Autodesk Inventor part; units mm, degrees
ref_plane "YZ Plane" through (0, 0, 0) normal (1, 0, 0) x (0, 1, 0)
ref_plane "XZ Plane" through (0, 0, 0) normal (0, 1, 0) x (-1, 0, 0)
ref_plane "XY Plane" through (0, 0, 0) normal (0, 0, 1) x (1, 0, 0)
sketch "Boceto1" plane through (0, 0, 0) normal (0, 0, 1) x (1, 0, 0)
  line L0 (220, 79) -> (220, 30)
  line L1 (229.5, 46) -> (229.5, 75)
  line L2 (235.5, 75) -> (235.5, 46)
  line L3 (229.5, -15) -> (229.5, 14)
  line L4 (235.5, 14) -> (235.5, -15)
  circle A0 centre (222.4918, -17.5) radius 1.6
  circle A1 centre (222.4918, 27.5) radius 1.6
  circle A2 centre (245.5, 27.5) radius 1.6
  circle A3 centre (245.5, -17.5) radius 1.6
  circle A4 centre (222.4918, 80) radius 1.6
  circle A5 centre (245.5, 75.9891) radius 1.6
  line L5 (220, 30) -> (220, -25)
  line L6 (229.5, 75) -> (230.4, 75)
  line L7 (231.4, 46) -> (229.5, 46)
  line L8 (220, -25) -> (227, -25)
  line L9 (238, -25) -> (240, -25)
  line L10 (231.4, -15) -> (229.5, -15)
  line L11 (229.5, 14) -> (231.4, 14)
  line L12 (230.4, 75) -> (235.5, 75)
  line L13 (231.4, 46) -> (235.5, 46)
  line L14 (231.4, 14) -> (235.5, 14)
  line L15 (231.4, -15) -> (235.5, -15)
  line L16 (227, -25) -> (238, -25)
  line L17 (245, 85) -> (220, 85)
  line L18 (220, 79) -> (220, 85)
  line L19 (251, 85) -> (251, -25)
  line L20 (240, -25) -> (251, -25)
  line L21 (245, 85) -> (251, 85)
  point P0 (0, 0)
  point P1 (245, -15)
  point P2 (245, 75)
  dimension "d2" = 6
  dimension "d3" = 9.5
  dimension "d4" = 6
  dimension "d5" = 9.5
  dimension "d6" = 29
  dimension "d9" = 9.0109
  dimension "d10" = 5
  dimension "d11" = 10
  dimension "d14" = 25.5
  dimension "d15" = 25.5
  dimension "d16" = 25.5
extrude "Extrusión1" add sketch "Boceto1" along normal blind 5
fillet "Empalme1" radius 1 2 edges at (251, 85, 2.5) (220, 85, 2.5)
fillet "Empalme2" radius 5 1 edges at (251, -25, 2.5)
properties part number "suplemento cojinete tapa"
Design review of the part built by this model. Coordinates are the model's own, in mm. A direction names the side the tool comes from. Give positions to 0.01 mm unless a question says otherwise; leave off trailing zeros. Write each loop counter-clockwise with the first axis right and the second up, starting at its lowest first coordinate (ties: lowest second). Pieces come first, ordered by that corner, then holes. Notation, with made-up numbers: M -33.5,22 L 3.5,22 A31 ccw 3.5,56 Z; hole C -1.75,30.5 d4. An arc over 180 degrees is marked long. Return JSON: item names as keys, results as strings. Group by question number.
Item 1: Take a section at A-A (y = 80). Give the boundary of the cut face in (x, z).
Item 2: Clearance check with a flat-ended pin moving along its axis: pin 1 Ø5 at (x, y) = (228, 17) entering from -Z. State where the tip first meets the part, or that it passes through.
Item 3: The part is to be moulded in two halves that separate along Y. For faces 3 (the flat face through (236, 85, 2)), 4 (the flat face through (232, 14, 2)), 5 (the flat face through (233, -25, 2)), say which applies: pulls with the +Y half, pulls with the -Y half, needs draft (parallel to the pull), parting line crosses it, or undercut.
Item 4: Tool access review of faces 1 (the flat face through (233, 46, 2)), 2 (the flat face through (220, 30, 2)): name each direction out of +Z, -Z, +X, -X, +Y, -Y from which nothing blocks a thin tool from reaching the whole face with its end or side.
Item 5: Wall thickness on line 1 along Y through (x, z) = (245.5, 2.95); line 2 along Y through (x, z) = (231, 0.75); line 3 along X through (y, z) = (-2, 0.65): over which ranges is each line inside the solid? List them lowest first.
Item 6: Take a section at C-C (z = 1.8). Count the separate pieces of the cut face and the enclosed holes in it, plus the area to 3 significant figures.
Item 7: Take a section at B-B (y = -17.5). Give the boundary of the cut face in (x, z).
Return value:
{
 "1": {"outline": "M 220,0 L 220.89,0 L 220.89,5 L 220,5 Z; M 224.09,0 L 251,0 L 251,5 L 224.09,5 Z"},
 "2": {"pin 1": "stops at z = 0"},
 "3": {"face 3": "pulls with the +Y half", "face 4": "undercut", "face 5": "pulls with the -Y half"},
 "4": {"face 1": "+Z, -Z", "face 2": "+Z, -Z, -X, +Y, -Y"},
 "5": {"line 1": "y = -25 to -19.1, -15.9 to 25.9, 29.1 to 74.39, 77.59 to 85", "line 2": "y = -25 to -15, 14 to 46, 75 to 85", "line 3": "x = 220 to 229.5, 235.5 to 251"},
 "6": {"separate pieces": "1", "enclosed holes": "8", "area": "3,010 mm2"},
 "7": {"outline": "M 220,0 L 220.89,0 L 220.89,5 L 220,5 Z; M 224.09,0 L 243.9,0 L 243.9,5 L 224.09,5 Z; M 247.1,0 L 251,0 L 251,5 L 247.1,5 Z"}
}
